Design review of the part built by this model. Coordinates are the model's own, in mm. Round coordinates to 2 decimals unless told otherwise and drop trailing zeros. Loops run counter-clockwise (first coordinate to the right, second up) from the corner with the lowest first, then second, coordinate; pieces in that order, holes last. Notation, with made-up numbers: (66, -11.5) -> (71, -11.5) arc R25 ccw to (71, 0.5) -> close; hole circle Ø3 at (63.5, 65.25). An arc over 180 degrees is marked (long way). Answer as CSV lines item,"result". Start each with the question number.
(1) For P1, Ø5, axis at x = 26, y = -4, coming from the -Z side; P2, Ø1, axis at x = 7.5, z = 1, coming from the -Y side; P3, Ø1, axis at y = 48, z = 1, coming from the -X side, all flat-tipped, find the tip position at first contact; note any pin that passes through.
(2) Take a section at D-D, the plane y = 74. Write out the cut boundary in (x, z), and give its area (3 significant figures).
(3) Take a section at C-C, the plane x = 57.15. Write out the cut boundary in (y, z).
(4) Take a section at B-B, the plane z = 1. State how many separate pieces and enclosed holes the cut face has, and give its area (3 significant figures).
(5) Take a section at A-A, the plane x = 28.5. Write out the cut boundary in (y, z), and give its area (3 significant figures).
(6) To check wall thickness, follow line 1 (Y direction, x = 21.5, z = 0.4); line 2 (X direction, y = -19, z = 1.3); line 3 (Y direction, x = 35, z = 0.35). State the ranges of each line that lie inside material, in increasing order. Write a range as from..to.
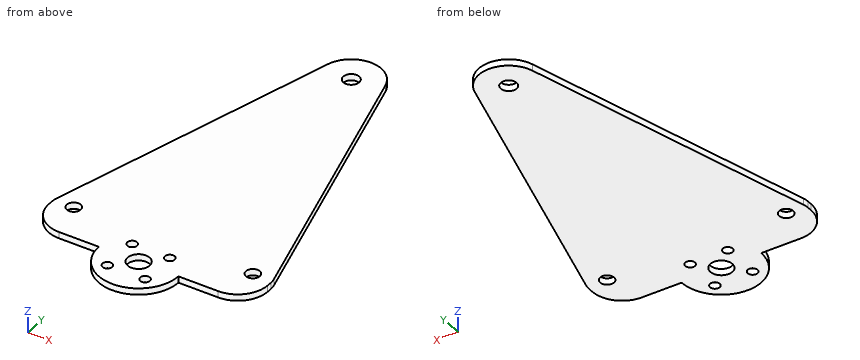
from build123d import *

# Parameters (mm, degrees)
SKETCH1_R           = 2.2225
SKETCH1_R_2         = 1.55
SKETCH1_R_3         = 2.539999998
SKETCH1_R_4         = 3.5
BOSS_EXTRUDE1_DEPTH = 2.032


with BuildPart() as part:
    # Sketch1 → Boss-Extrude1 (new body)
    with BuildSketch(Plane.XY):
        with BuildLine():
            Line((41.275, -11.969713646), (53.975, -11.969713646))
            ThreePointArc((53.975, -11.969713646), (60.710192091, -9.179905737), (63.5, -2.444713646))
            Line((63.5, -2.444713646), (63.5, -0.857213646))
            ThreePointArc((63.5, -0.857213646), (63.442919511, -0.007705539), (63.272704244, 0.826530021))
            Line((63.272704244, 0.826530021), (37.759056366, 93.603431401))
            ThreePointArc((37.759056366, 93.603431401), (28.575, 100.6028159), (19.390943634, 93.603431401))
            Line((19.390943634, 93.603431401), (-6.122704244, 0.826530021))
            ThreePointArc((-6.122704244, 0.826530021), (-6.292919511, -0.007705539), (-6.35, -0.857213646))
            Line((-6.35, -0.857213646), (-6.35, -2.444713646))
            ThreePointArc((-6.35, -2.444713646), (-3.560192091, -9.179905737), (3.175, -11.969713646))
            Line((3.175, -11.969713646), (15.875, -11.969713646))
            ThreePointArc((15.875, -11.969713646), (28.575, -24.669713646), (41.275, -11.969713646))
        make_face()
        Circle(SKETCH1_R, mode=Mode.SUBTRACT)
        with Locations((57.15, 0)):
            Circle(SKETCH1_R, mode=Mode.SUBTRACT)
        with Locations((22.56459236, -5.959306006)):
            Circle(SKETCH1_R_2, mode=Mode.SUBTRACT)
        with Locations((28.575, 91.0778159)):
            Circle(SKETCH1_R_3, mode=Mode.SUBTRACT)
        with Locations((28.575, -11.969713646)):
            Circle(SKETCH1_R_4, mode=Mode.SUBTRACT)
        with Locations((34.58540764, -17.980121287)):
            Circle(SKETCH1_R_2, mode=Mode.SUBTRACT)
        with Locations((34.58540764, -5.959306006)):
            Circle(SKETCH1_R_2, mode=Mode.SUBTRACT)
        with Locations((22.56459236, -17.980121287)):
            Circle(SKETCH1_R_2, mode=Mode.SUBTRACT)
    extrude(amount=BOSS_EXTRUDE1_DEPTH)


solid = part.part
The answers:
1,P1,"z = 0"
1,P2,"y = -11.97"
1,P3,"x = 6.71"
2,outline,"(14, 0) -> (43.15, 0) -> (43.15, 2.03) -> (14, 2.03) -> close"
2,area,"59.2 mm²"
3,outline,"(-11.42, 0) -> (-2.22, 0) -> (-2.22, 2.03) -> (-11.42, 2.03) -> close; (2.22, 0) -> (23.09, 0) -> (23.09, 2.03) -> (2.22, 2.03) -> close"
4,separate pieces,"1"
4,enclosed holes,"8"
4,area,"5,150 mm²"
5,outline,"(-24.67, 0) -> (-15.47, 0) -> (-15.47, 2.03) -> (-24.67, 2.03) -> close; (-8.47, 0) -> (88.54, 0) -> (88.54, 2.03) -> (-8.47, 2.03) -> close; (93.62, 0) -> (100.6, 0) -> (100.6, 2.03) -> (93.62, 2.03) -> close"
5,area,"230 mm²"
6,line 1,"-22.52..-19.11, -16.85..-7.09, -4.83..97.46"
6,line 2,"18..21.4, 23.73..33.42, 35.75..39.15"
6,line 3,"-22.92..-19.47, -16.49..-7.45, -4.47..98.11"
